Geometry check sheet. Reference: the model listing, model coordinates, mm. Face numbers are marked on the shaded views. A direction names the side the tool comes from. Round coordinates to 2 decimals unless told otherwise and drop trailing zeros. Loops run counter-clockwise (first coordinate to the right, second up) from the corner with the lowest first, then second, coordinate; pieces in that order, holes last. Notation, with made-up numbers: M 89,-6 L 99,-6 A16 cw 99,13 Z; hole C 25.25,-28 d1. An arc over 180 degrees is marked long. Use one line per item in the form item = value. Start each with the question number.
1. Draft check along X on the marked faces 1, 2 and 3. Enter one of: pulls with the +X half, pulls with the -X half, needs draft (parallel to the pull), parting line crosses it, or undercut.
2. Cross-section at A-A (y = 0). Record the boundary of the cut face in (x, z).
3. Cross-section at C-C (x = 0). Record the boundary of the cut face in (y, z).
4. Material ranges on line 1 (Z direction, x = -5, y = 4); line 2 (X direction, y = -6.5, z = 5); line 3 (Y direction, x = 2.5, z = 3.75), recorded low to high.
5. Cross-section at B-B (z = 6.5). Record the boundary of the cut face in (x, y).
6. Set-up check for the marked faces 4, 5, 6, 7 and 8: record each of +Z, -Z, +X, -X, +Y, -Y from which the full face is reachable in a straight line by a thin tool's end or side.
7. Go/stop test with flat-tipped pins: pin 1 (1.5 mm diameter, centred on y = -3.5, z = 9.5, fed in from +X); pin 2 (2 mm diameter, centred on x = -4.5, z = 6.5, fed in from +Y); pin 3 (12 mm diameter, centred on x = -7.5, y = 8, fed in from +Z); pin 4 (6 mm diameter, centred on x = 3.5, y = -2, fed in from +Z). Record where each tip stops, or that it passes through.
8. Cross-section at D-D (z = 1.25). Record the boundary of the cut face in (x, y), then the cut area to 3 significant figures.
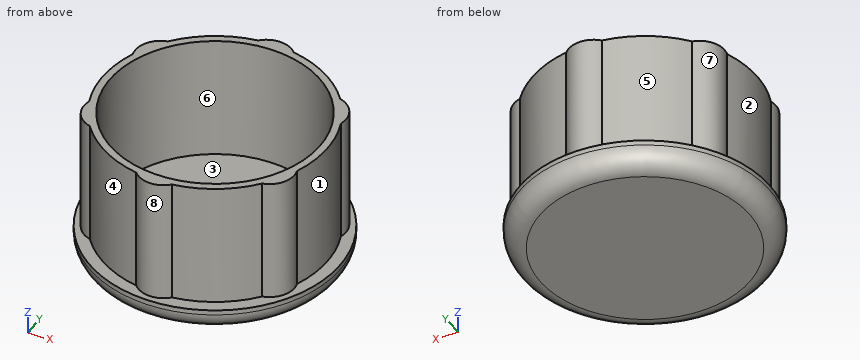
```python
from build123d import *

# Parameters (mm, degrees)
F0_R            = 10
F1_DEPTH        = 2
F2_R            = 1.6
F4_R            = 9
F4_R_2          = 8.4
F5_DEPTH        = 10
F7_DEPTH        = 10
F7_COPIES_COUNT = 6


# Not quite as in the source:
# - a pattern or mirror of a feature is missing from the dataset's text; its kind, count and spacing are read off the source's solid


with BuildPart() as f1:
    # F0 (on Top) → F1 (new body)
    with BuildSketch(Plane.XY):
        Circle(F0_R)
    extrude(amount=F1_DEPTH)

    # F2
    f2_edges = [f1.edges().sort_by_distance(p)[0] for p in [
        (-10, 0, 0),
    ]]
    fillet(f2_edges, radius=F2_R)

    # F4 (on face) → F5 (join)
    with BuildSketch(Plane.XY.offset(2)):
        Circle(F4_R)
        Circle(F4_R_2, mode=Mode.SUBTRACT)
    extrude(amount=F5_DEPTH)

    # F6 (on face) → F7 (join, through all)
    with BuildSketch(Plane.XY.offset(2)):
        with BuildLine():
            ThreePointArc((-1.4444337606, 8.8833333333), (0, 9), (1.4444337606, 8.8833333333))
            ThreePointArc((1.4444337606, 8.8833333333), (0, 9.5), (-1.4444337606, 8.8833333333))
        make_face()
    f7 = extrude(amount=F7_DEPTH)

    # F7_copies: F7 ×6 about axis
    f7_copies_axis = Axis((0, 0, 0), (0, 0, 1))
    for i in range(1, F7_COPIES_COUNT):
        add(f7.rotate(f7_copies_axis, i * 360 / F7_COPIES_COUNT))


solid = f1.part
```
Reported:
q1.face_1 = pulls with the +X half
q1.face_2 = pulls with the -X half
q1.face_3 = undercut
q2.outline = M -10,1.6 A1.6 ccw -8.4,0 L 8.4,0 A1.6 ccw 10,1.6 L 10,2 L 9,2 L 9,12 L 8.4,12 L 8.4,2 L -8.4,2 L -8.4,12 L -9,12 L -9,2 L -10,2 Z
q3.outline = M -10,1.6 A1.6 ccw -8.4,0 L 8.4,0 A1.6 ccw 10,1.6 L 10,2 L 9.5,2 L 9.5,12 L 8.4,12 L 8.4,2 L -8.4,2 L -8.4,12 L -9.5,12 L -9.5,2 L -10,2 Z
q4.line_1 = 0 to 2
q4.line_2 = -6.22 to -5.32, 5.32 to 6.22
q4.line_3 = -8.65 to -8.02, 8.02 to 8.65
q5.outline = M -8.42,-3.19 A2 ccw -6.97,-5.69 A9 ccw -1.44,-8.88 A2 ccw 1.44,-8.88 A9 ccw 6.97,-5.69 A2 ccw 8.42,-3.19 A9 ccw 8.42,3.19 A2 ccw 6.97,5.69 A9 ccw 1.44,8.88 A2 ccw -1.44,8.88 A9 ccw -6.97,5.69 A2 ccw -8.42,3.19 A9 ccw Z; hole C 0,0 d16.8
q6.face_4 = +Z, -X, -Y
q6.face_5 = +Z, -X, +Y
q6.face_6 = +Z
q6.face_7 = +Z, -X
q6.face_8 = +Z, -Y
q7.pin_1 = 8.57
q7.pin_2 = 8.29
q7.pin_3 = 12
q7.pin_4 = 2
q8.outline = C 0,0 d19.92
q8.area = 312 mm²
